Input: part model. Units: mm. Frame: model coordinates. A direction names the side the tool comes from. Coordinates: 2 decimals unless noted, no trailing zeros. Loops run counter-clockwise (first coordinate to the right, second up) from the corner with the lowest first, then second, coordinate; pieces in that order, holes last. Notation, with made-up numbers: (-32, 61.5) - (5, 61.5) arc R25 cw to (5, 92.5) - close; hole circle Ø3 at (87, 28). An arc over 180 degrees is marked (long way). Use one line per item in the form item = value.
from build123d import *

# Parameters (mm, degrees)
F0_R          = 4
F1_DEPTH      = 8
F1_DEPTH_BACK = 80
F0_R_2        = 5
F2_DEPTH      = 80
F3_R          = 3
F4_DEPTH      = 17
F5_SIZE       = 1
F6_SIZE       = 0.5


with BuildPart() as f1:
    # F0 (on Top) → F1 (new body, two sides)
    with BuildSketch(Plane.XY) as f1_sk:
        Circle(F0_R)
    extrude(amount=F1_DEPTH)
    extrude(f1_sk.sketch, amount=-F1_DEPTH_BACK)



with BuildPart() as f2:
    # F0 (on Top) → F2 (new body)
    with BuildSketch(Plane.XY):
        Circle(F0_R_2)
        Circle(F0_R, mode=Mode.SUBTRACT)
    extrude(amount=-F2_DEPTH)


with BuildPart() as f1_1:
    add(f1.part)

    add(f2.part)  # F4 merges F2
    # F3 (on Front) → F4 (join)
    with BuildSketch(Plane.XZ):
        with Locations((0, -12)):
            Circle(F3_R)
    extrude(amount=F4_DEPTH)

    # F5
    f5_edges = [f1_1.edges().sort_by_distance(p)[0] for p in [
        (-5, 0, -80),
        (-4, 0, 8),
    ]]
    chamfer(f5_edges, length=F5_SIZE)

    # F6
    f6_edges = [f1_1.edges().sort_by_distance(p)[0] for p in [
        (-3, -17, -12),
    ]]
    chamfer(f6_edges, length=F6_SIZE)


solid = f1_1.part
Q1. Set-up query: faces 1 (the cylindrical face through (-3, -10, -12)), 2 (the flat face through (0, 0, 8)), 3 (the cylindrical face through (-0.867, -3.905, 3.549)). Return all of +Z, -Z, +X, -X, +Y, -Y with unobstructed straight access to the full face (end or side cutting, diameter ignored); none if empty.
Check values:
face_1 = -Y
face_2 = +Z, +X, -X, +Y, -Y
face_3 = +Z
Q2. Cut plane C-C, the plane y = 0. Return loops of the section in (x, z), then the cut area to 3 significant figures.
Check values:
outline = (-5, -79) - (-4, -80) - (4, -80) - (5, -79) - (5, 0) - (4, 0) - (4, 7) - (3, 8) - (-3, 8) - (-4, 7) - (-4, 0) - (-5, 0) - close
area = 862 mm²
Q3. Ray query, line 1 along Y through (x, z) = (-3, -75); line 2 along Y through (x, z) = (-1, -1); line 3 along Z through (x, y) = (-0.25, -9.5). Return the intervals inside material, ascending. Write a range as [from, to].
Check values:
line_1 = [-4, 4]
line_2 = [-4.9, 4.9]
line_3 = [-14.99, -9.01]
Q4. Cut plane B-B, the plane x = 0. Return loops of the section in (y, z).
Check values:
outline = (-17, -14.5) - (-16.5, -15) - (-5, -15) - (-5, -79) - (-4, -80) - (4, -80) - (5, -79) - (5, 0) - (4, 0) - (4, 7) - (3, 8) - (-3, 8) - (-4, 7) - (-4, 0) - (-5, 0) - (-5, -9) - (-16.5, -9) - (-17, -9.5) - close
Q5. Cut plane A-A, the plane z = -12. Return loops of the section in (x, y).
Check values:
outline = (-3, -16.5) - (-2.5, -17) - (2.5, -17) - (3, -16.5) - (3, -4) arc R5 ccw (long way) to (-3, -4) - close
Q6. First-contact query: P1, Ø12, axis at y = -4.5, z = -27, coming from the +X side; P2, Ø1, axis at x = 3, y = -14.5, coming from the -Z side; P3, Ø1.5, axis at x = -0.5, z = -25.5, coming from the -Y side; P4, Ø1.5, axis at x = 1, y = -13, coming from the -Z side. Flat tips, straight axial feed; report the tip coordinate or a pass-through.
Check values:
P1 = 5
P2 = -13.66
P3 = -5
P4 = -14.99
Q7. Cut plane D-D, the plane z = -1.5. Return loops of the section in (x, y), then the cut area to 3 significant figures.
Check values:
outline = circle Ø10 at (0, 0)
area = 78.5 mm²
